Check sheet for the modelled part. Datum: model origin and axes. Units: mm. Face numbers are marked on the shaded views. A direction names the side the tool comes from. Round coordinates to 2 decimals unless told otherwise and drop trailing zeros. Loops run counter-clockwise (first coordinate to the right, second up) from the corner with the lowest first, then second, coordinate; pieces in that order, holes last. Notation, with made-up numbers: (-34.5, 14) - (21.5, 14) arc R9 ccw to (21.5, 26) - close; hole circle Ø3 at (-8.75, 43.5). An arc over 180 degrees is marked (long way). Put each result on its own line as item: value. Start each with the question number.
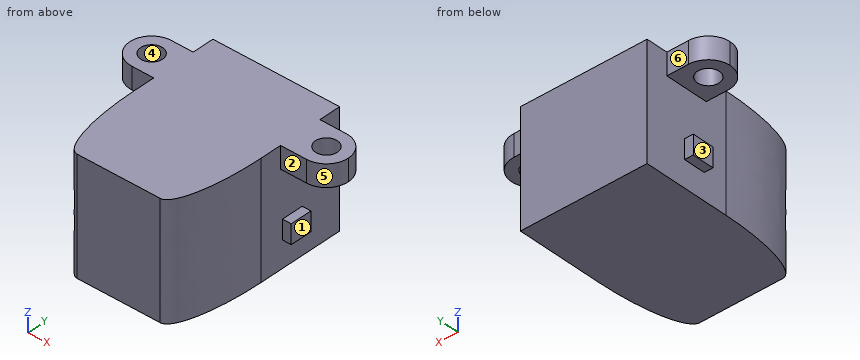
```python
from build123d import *

# Parameters (mm, degrees)
SKETCH1_W                = 29
SKETCH1_H                = 40
BOSS_EXTRUDE1_DEPTH      = 26.2
FILLET1_SIZE             = 20
FILLET1_SIZE_2           = 5
BOSS_EXTRUDE2_DEPTH      = 10
BOSS_EXTRUDE2_DEPTH_BACK = 40
SKETCH5_W                = 5
SKETCH5_H                = 10
FILLET2_R                = 5
SKETCH6_R                = 2.5
CUT_EXTRUDE2_DEPTH       = 6
BOSS_EXTRUDE3_DEPTH      = 2
BOSS_EXTRUDE3_DEPTH_BACK = 31


# Some blends are built 0.0001 mm under size
with BuildPart() as part:
    # Sketch1 → Boss-Extrude1 (new body)
    with BuildSketch(Plane.XY):
        with Locations((14.5, -20)):
            Rectangle(SKETCH1_W, SKETCH1_H)
    extrude(amount=BOSS_EXTRUDE1_DEPTH)

    # Fillet1
    # an asymmetric fillet: 20, 5 mm, written as the material it takes off along each edge
    with BuildSketch(Plane(origin=(29, -40, -50), x_dir=(0, 1, 0), z_dir=(0, 0, 1))) as fillet1_piece_1:
        with BuildLine():
            Bezier((FILLET1_SIZE, 0), (0, 0), (0, FILLET1_SIZE_2), weights=[1, 0.707106781, 1])
            Line((0, FILLET1_SIZE_2), (0, 0))
            Line((0, 0), (FILLET1_SIZE, 0))
        make_face()
    extrude(amount=126.2, mode=Mode.SUBTRACT)
    with BuildSketch(Plane(origin=(0, -40, -50), x_dir=(1, 0, 0), z_dir=(0, 0, 1))) as fillet1_piece_2:
        with BuildLine():
            Bezier((FILLET1_SIZE_2, 0), (0, 0), (0, FILLET1_SIZE), weights=[1, 0.707106781, 1])
            Line((0, FILLET1_SIZE), (0, 0))
            Line((0, 0), (FILLET1_SIZE_2, 0))
        make_face()
    extrude(amount=126.2, mode=Mode.SUBTRACT)

    # Sketch5 → Boss-Extrude2 (add, two sides: drawn at the far end of the back side and taken through both)
    with BuildSketch(Plane.ZY.offset(-BOSS_EXTRUDE2_DEPTH_BACK)):
        with Locations((23.7, -10)):
            Rectangle(SKETCH5_W, SKETCH5_H)
    extrude(amount=BOSS_EXTRUDE2_DEPTH + BOSS_EXTRUDE2_DEPTH_BACK)

    # Fillet2
    fillet2_edges = [part.edges().sort_by_distance(p)[0] for p in [
        (40, -15, 23.7),
        (40, -5, 23.7),
        (-10, -15, 23.7),
        (-10, -5, 23.7),
    ]]
    fillet(fillet2_edges, radius=FILLET2_R - 0.0001)  # a hair under: the kernel refuses the full size

    # Sketch6 → Cut-Extrude2 (cut)
    with BuildSketch(Plane.XY.offset(26.2)):
        with Locations((-5, -10)):
            Circle(SKETCH6_R)
        with Locations((35, -10)):
            Circle(SKETCH6_R)
    extrude(amount=-CUT_EXTRUDE2_DEPTH, mode=Mode.SUBTRACT)

    # Sketch7 → Boss-Extrude3 (add, two sides: drawn at the far end of the back side and taken through both)
    with BuildSketch(Plane(origin=(29, 0, 0), x_dir=(0, 0, -1), z_dir=(1, 0, 0)).offset(-BOSS_EXTRUDE3_DEPTH_BACK)):
        Polygon((-8.2, -9.5), (-6, -9.5), (-6, -12), (-6, -14.5), (-8.2, -14.5), (-10.4, -14.5), (-10.4, -12), (-10.4, -9.5), align=None)
    extrude(amount=BOSS_EXTRUDE3_DEPTH + BOSS_EXTRUDE3_DEPTH_BACK)


solid = part.part
```
Q1. Cross-section at A-A on y = -18. Enter the section's corners in (x, z).
Q2. Set-up check for the marked faces 1, 2 and 3: record each of +Z, -Z, +X, -X, +Y, -Y from which the full face is reachable in a straight line by a thin tool's end or side.
Q3. Draft check along X on the marked faces 4, 5 and 6. Enter one of: +X half, -X half, draft (parallel to the pull), parting line (faces both ways), or undercut.
Q4. Material ranges on line 1 (Y direction, x = -5, z = 22.4); line 2 (X direction, y = -9.5, z = 22.5); line 3 (X direction, y = -3, z = 20), recorded low to high. Write a range as from..to.
Q5. Depth check by flat-ended pin: pin 1 Ø3 at (y, z) = (-9.5, 15) entering from -X; pin 2 Ø5 at (y, z) = (-25.5, 10) entering from +X; pin 3 Ø5 at (y, z) = (-11, 9) entering from -X. Enter the tip coordinate at first touch or a pass-through.
Answer list:
1. outline: (0, 0) - (29, 0) - (29, 26.2) - (0, 26.2) - close
2. face 1: -Z, +X, +Y, -Y
2. face 2: +Z, -Z, +X, -Y
2. face 3: -Z, -X, +Y, -Y
3. face 4: undercut
3. face 5: +X half
3. face 6: draft
4. line 1: y = -15..-12.5, -7.5..-5
4. line 2: x = -9.97..-7.45, -2.55..32.55, 37.45..39.97
4. line 3: x = 0..29
5. pin 1: stops at x = 0
5. pin 2: stops at x = 28.94
5. pin 3: stops at x = -2
